Geometry check sheet. Reference: the model listing, model coordinates, mm. A direction names the side the tool comes from. Coordinates: 2 decimals unless noted, no trailing zeros. Write each loop counter-clockwise with the first axis right and the second up, starting at its lowest first coordinate (ties: lowest second). Pieces come first, ordered by that corner, then holes. Notation, with made-up numbers: (55, -4.75) - (97, -4.75) arc R26 ccw to (97, 17.25) - close; hole circle Ø3 at (87.25, -24). An arc over 180 degrees is marked (long way). Answer as a JSON object with one key per item and string values. Group by question number.
from build123d import *

# Parameters (mm, degrees)
SKETCH_R      = 25.898575
PAD_DEPTH     = 12.4
SKETCH001_R   = 19.464616
SKETCH001_R_2 = 10
PAD001_DEPTH  = 20.5
SKETCH002_R   = 17
PAD002_DEPTH  = 13


with BuildPart() as part:
    # Sketch → Pad (new body)
    with BuildSketch(Plane.XY):
        Circle(SKETCH_R)
        Polygon((8.12282, 14.039523), (-8.097173, 14.05433), (-16.219993, 0.014807), (-8.12282, -14.039523), (8.097173, -14.05433), (16.219993, -0.014807), align=None, mode=Mode.SUBTRACT)
    extrude(amount=PAD_DEPTH)

    # Sketch001 (on Face9 of Pad) → Pad001 (join)
    with BuildSketch(Plane.XY.offset(12.4)):
        Circle(SKETCH001_R)
        Circle(SKETCH001_R_2, mode=Mode.SUBTRACT)
    extrude(amount=PAD001_DEPTH)

    # Sketch002 (on Face12 of Pad001) → Pad002 (join)
    with BuildSketch(Plane.XY.offset(32.9)):
        Circle(SKETCH002_R)
        Polygon((-7.484853, 5.915115), (-8.865066, -3.524515), (-1.380213, -9.43963), (7.484853, -5.915115), (8.865066, 3.524515), (1.380213, 9.43963), align=None, mode=Mode.SUBTRACT)
    extrude(amount=PAD002_DEPTH)


solid = part.part
(1) Section check C-C (y = -1). Record the cut outline in (x, z).
(2) Section check D-D (z = 27). Record the cut outline in (x, y), and give its area (3 significant figures).
(3) Gauge pin test, flat ends, axial feed: pin 1 (10 mm diameter, centred on x = -2, z = 19, fed in from +Y); pin 2 (6 mm diameter, centred on y = 14.5, z = 26, fed in from +X); pin 3 (4 mm diameter, centred on x = 11, z = 15, fed in from +Y). Record the tip position at first contact, or that the pin passes through.
(4) Draft check along X on faces 1 (the face through (4, 8, 45.9)), 2 (the face through (-12.23, -6.91, 6.11)), 3 (the face through (-25.874, 1.139, 6.113)). Enter one of: +X half, -X half, draft (parallel to the pull), parting line (faces both ways), or undercut.
(5) Section check A-A (x = 0). Record the cut outline in (y, z), and give its area (3 significant figures).
(6) Material ranges on L1, parallel to Y at x = 0, z = 24.75; L2, parallel to Z at x = -20, y = 2.5; L3, parallel to X at y = -5, z = 15, recorded low to high. Write a range as [from, to].
(7) Section check B-B (z = 5). Record the cut outline in (x, y), and give its area (3 significant figures).
(8) Set-up check for faces 4 (the face through (5.175, 6.441, 39.309)), 5 (the face through (3, 10, 12.4)), 6 (the face through (11, -11, 0)), 7 (the face through (18.566, 5.847, 22.507)): record each of +Z, -Z, +X, -X, +Y, -Y from which the full face is reachable in a straight line by a thin tool's end or side.
Conclusion:
{
 "1": {"outline": "(-25.88, 0) - (-15.64, 0) - (-15.64, 12.4) - (-9.95, 12.4) - (-9.95, 32.9) - (-8.5, 32.9) - (-8.5, 45.9) - (-16.97, 45.9) - (-16.97, 32.9) - (-19.44, 32.9) - (-19.44, 12.4) - (-25.88, 12.4) - close; (8.2, 32.9) - (9.95, 32.9) - (9.95, 12.4) - (15.65, 12.4) - (15.65, 0) - (25.88, 0) - (25.88, 12.4) - (19.44, 12.4) - (19.44, 32.9) - (16.97, 32.9) - (16.97, 45.9) - (8.2, 45.9) - close"},
 "2": {"outline": "circle Ø38.93 at (0, 0); hole circle Ø20 at (0, 0)", "area": "876 mm^2"},
 "3": {"pin 1": "stops at y = 19.46", "pin 2": "stops at x = 15.7", "pin 3": "stops at y = 17.26"},
 "4": {"face 1": "draft", "face 2": "undercut", "face 3": "parting line"},
 "5": {"outline": "(-25.9, 0) - (-14.05, 0) - (-14.05, 12.4) - (-10, 12.4) - (-10, 32.9) - (-8.89, 32.9) - (-8.89, 45.9) - (-17, 45.9) - (-17, 32.9) - (-19.46, 32.9) - (-19.46, 12.4) - (-25.9, 12.4) - close; (8.89, 32.9) - (10, 32.9) - (10, 12.4) - (14.05, 12.4) - (14.05, 0) - (25.9, 0) - (25.9, 12.4) - (19.46, 12.4) - (19.46, 32.9) - (17, 32.9) - (17, 45.9) - (8.89, 45.9) - close", "area": "893 mm^2"},
 "6": {"L1": "y = [-19.46, -10], [10, 19.46]", "L2": "z = [0, 12.4]", "L3": "x = [-18.81, -8.66], [8.66, 18.81]"},
 "7": {"outline": "circle Ø51.8 at (0, 0); hole (-16.22, 0.01) - (-8.12, -14.04) - (8.1, -14.05) - (16.22, -0.01) - (8.12, 14.04) - (-8.1, 14.05) - close", "area": "1,420 mm^2"},
 "8": {"face 4": "+Z, -Z", "face 5": "-Z", "face 6": "-Z, +X, -X, +Y, -Y", "face 7": "+Z"}
}
